Can you work these out from the drawing? Everything is in mm from the part's minimum corner. A direction names the side the tool comes from. Round coordinates to 2 decimals unless told otherwise and drop trailing zeros. Order: outer loops, then holes, each group sorted by start corner. A loop starts at its lowest first (then second) coordinate and runs counter-clockwise, first axis right, second up. Notation, with made-up numbers: (-25.75, -31) -> (10.25, -31) arc R16 ccw to (10.25, -8) -> close; hole circle Ø9 at (-37.75, 51). An arc over 180 degrees is marked (long way). One line per item, written item: value.
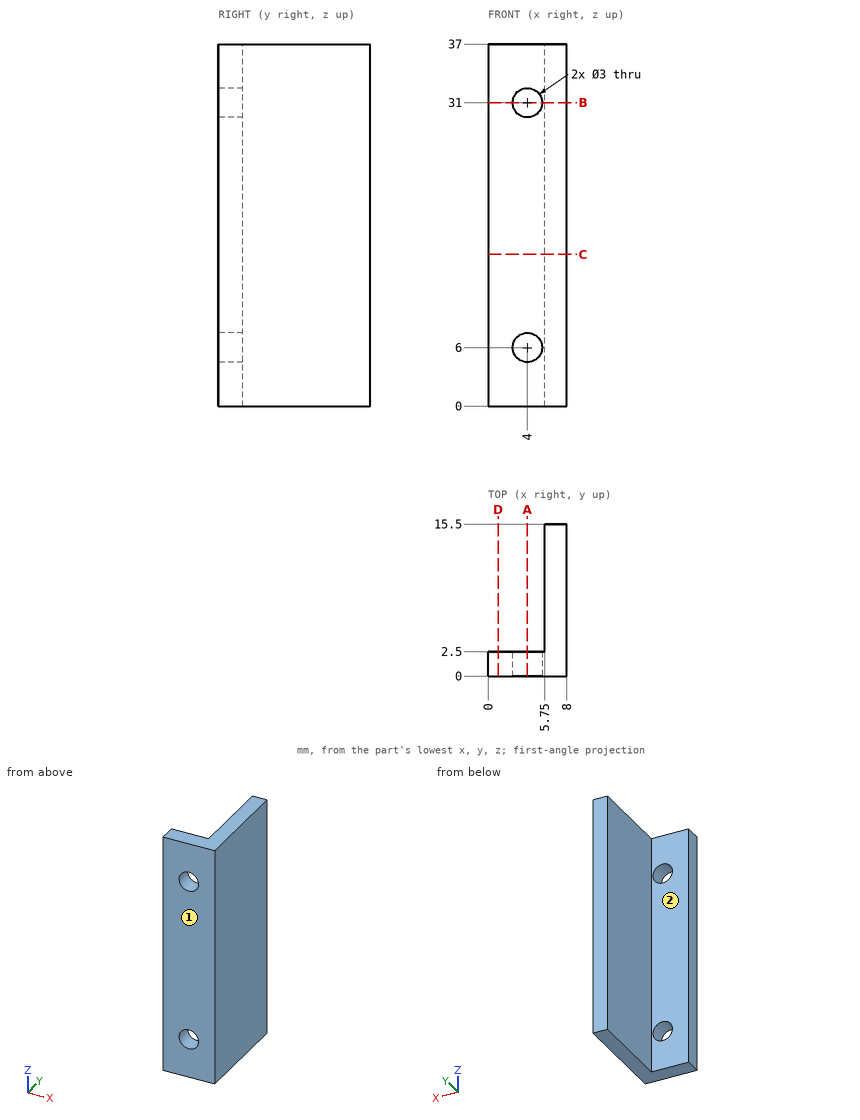
Q1. I need wall thicknesses on line 1 along Z through (x, y) = (4, 0.7); line 2 along Z through (x, y) = (3, 1.25); line 3 along Y through (x, z) = (1.25, 29.5). Which ranges of each line are inside material? Lowest first, please.
Answers:
line 1: 0 to 4.5, 7.5 to 29.5, 32.5 to 37
line 2: 0 to 4.88, 7.12 to 29.88, 32.12 to 37
line 3: 0 to 2.5
Q2. I want a section at B-B on z = 31. Write out the boundary of the cut face in (x, y), then the cut area to 4 significant figures.
Answers:
outline: (0, 0) -> (2.5, 0) -> (2.5, 2.5) -> (0, 2.5) -> close; (5.5, 0) -> (8, 0) -> (8, 15.5) -> (5.75, 15.5) -> (5.75, 2.5) -> (5.5, 2.5) -> close
area: 41.75 mm2
Q3. Which directions (+Z, -Z, +X, -X, +Y, -Y) give clear straight access to the entire face, cutting with the end or side of a thin tool? Please do the marked faces 1 and 2.
Answers:
face 1: +Z, -Z, +X, -X, -Y
face 2: +Z, -Z, -X, +Y
Q4. For P1, Ø3, axis at x = 2.5, z = 26.5, coming from the +Y side; P2, Ø8, axis at y = 9.5, z = 8.5, coming from the -X side, each with a flat end and sliding along its axis, tell me the tip position at first contact or that it passes through.
Answers:
P1: y = 2.5
P2: x = 5.75
Q5. I want a section at D-D on x = 1. Write out the boundary of the cut face in (y, z), then the cut area to 3 significant figures.
Answers:
outline: (0, 0) -> (2.5, 0) -> (2.5, 37) -> (0, 37) -> close
area: 92.5 mm2
Q6. I want a section at C-C on z = 15.5. Write out the boundary of the cut face in (x, y), then the cut area to 4 significant figures.
Answers:
outline: (0, 0) -> (8, 0) -> (8, 15.5) -> (5.75, 15.5) -> (5.75, 2.5) -> (0, 2.5) -> close
area: 49.25 mm2
Q7. I want a section at A-A on x = 4. Write out the boundary of the cut face in (y, z).
Answers:
outline: (0, 0) -> (2.5, 0) -> (2.5, 4.5) -> (0, 4.5) -> close; (0, 7.5) -> (2.5, 7.5) -> (2.5, 29.5) -> (0, 29.5) -> close; (0, 32.5) -> (2.5, 32.5) -> (2.5, 37) -> (0, 37) -> close
